Input: part model. Units: mm. Frame: model coordinates. Face numbers are marked on the shaded views. Give positions to 0.01 mm unless a question says otherwise; leave off trailing zeros. Loops run counter-clockwise (first coordinate to the right, second up) from the corner with the lowest first, then second, coordinate; pieces in that order, holes last. Notation, with made-up numbers: (61, 73) - (105, 73) arc R11 ccw to (105, 89) - close; hole circle Ø7 at (-7.75, 47.5). An arc over 180 degrees is marked (long way). One line per question, with ' | ' between items. Start each with the question number.
from build123d import *

# Parameters (mm, degrees)
SKETCH1_R               = 1.5
BOSS_EXTRUDE1_DEPTH     = 20
CUT_EXTRUDE1_DEPTH      = 21.315038789
CUT_EXTRUDE1_DEPTH_BACK = 21.315038789
SKETCH4_R               = 2.52
SKETCH4_R_2             = 1.25
CUT_EXTRUDE2_DEPTH      = 8
CHAMFER1_SIZE           = 0.25


with BuildPart() as part:
    # Sketch1 → Boss-Extrude1 (new body)
    with BuildSketch(Plane(origin=(0, 0, 0), x_dir=(1, 0, 0), z_dir=(0, 1, 0))):
        with Locations(Location((0, 0, 0), (0, 0, 270))):
            Circle(SKETCH1_R)
    extrude(amount=BOSS_EXTRUDE1_DEPTH)

    # Sketch2 → Revolve1 (revolve)
    with BuildSketch(Plane.XY, mode=Mode.PRIVATE) as revolve1_sk:
        with BuildLine():
            Line((0, 0), (-2.52, 0))
            ThreePointArc((-2.52, 0), (-1.585449748, -1.440539697), (0, -2.1))
            Line((0, -2.1), (0, 0))
        make_face()
    revolve(revolve1_sk.sketch.rotate(Axis((0, -2.1, 0), (0, 1, 0)), 180), axis=Axis((0, -2.1, 0), (0, 1, 0)))

    # Sketch3 → Cut-Extrude1 (cut, two sides: drawn at the far end of the back side and taken through both)
    with BuildSketch(Plane.XY.offset(-CUT_EXTRUDE1_DEPTH_BACK)):
        Polygon((-0.5, -0.7), (0, -0.7), (0.5, -0.7), (0.5, -4.6380618), (-0.5, -4.6380618), align=None)
    extrude(amount=CUT_EXTRUDE1_DEPTH + CUT_EXTRUDE1_DEPTH_BACK, mode=Mode.SUBTRACT)

    # Sketch4 → Cut-Extrude2 (cut)
    with BuildSketch(Plane(origin=(0, 0, 0), x_dir=(1, 0, 0), z_dir=(0, 1, 0))):
        Circle(SKETCH4_R)
        with Locations(Location((0, 0, 0), (0, 0, 180))):
            Circle(SKETCH4_R_2, mode=Mode.SUBTRACT)
    extrude(amount=CUT_EXTRUDE2_DEPTH, mode=Mode.SUBTRACT)

    # Chamfer1
    chamfer1_edges = [part.edges().sort_by_distance(p)[0] for p in [
        (0, 8, -1.5),
        (0, 20, -1.5),
    ]]
    chamfer(chamfer1_edges, length=CHAMFER1_SIZE - 0.0001)  # a hair under: the kernel refuses the full size


solid = part.part
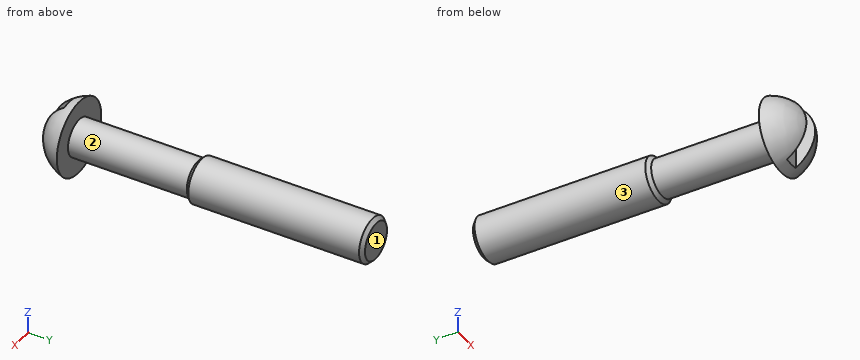
Q1. Line query: L1, parallel to Y at x = -0.35, z = 1; L2, parallel to Y at x = -0.1, z = -1.75; L3, parallel to Z at x = 0, y = 11.5. Output: solid intervals per line, ascending. Write a range as from..to.
Q2. First-contact query: pin 1 (3 mm diameter, centred on y = 4.5, z = 1.5, fed in from +X); pin 2 (0.7 mm diameter, centred on y = -1.5, z = -1, fed in from +X); pin 3 (0.8 mm diameter, centred on x = 0, z = 0.5, fed in from -Y). Flat tips, straight axial feed; report the tip coordinate or a pass-through.
Q3. Section A-A, the plane y = 4.75. Output: boundary loops of the cut face in (x, z).
Q4. Section B-B, the plane y = 15.5. Output: boundary loops of the cut face in (x, z), plus the area to 3 significant figures.
Q5. Draft query along Y for the marked faces 1, 2 and 3. Return one class per face: +Y half, -Y half, draft (parallel to the pull), parting line (faces both ways), or undercut.
Solved:
1) L1: y = -0.7..20 | L2: y = -0.7..0 | L3: z = -1.5..1.5
2) pin 1: stops at x = 1.25 | pin 2: stops at x = 1.65 | pin 3: stops at y = -0.7
3) outline: circle Ø2.5 at (0, 0)
4) outline: circle Ø3 at (0, 0) | area: 7.07 mm²
5) face 1: +Y half | face 2: undercut | face 3: draft
